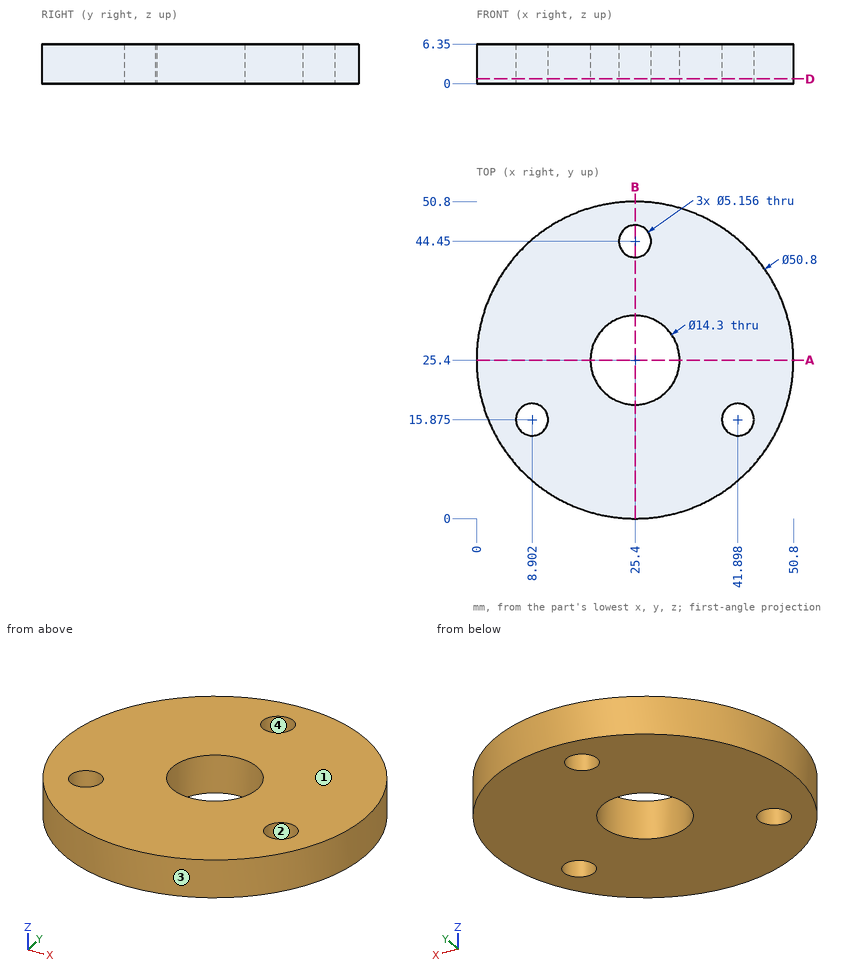
Job drawing, mm, ordinate dimensions from the low corner. One solid piece. Give positions to 0.01 mm unless a question says otherwise; leave off trailing zeros. Order: outer loops, then holes, each group sorted by start corner. A loop starts at its lowest first (then second) coordinate and runs counter-clockwise, first axis right, second up. Notation, with made-up numbers: M -8,59.25 L 25,59.25 A35 cw 25,96.25 Z; hole C 3,75 d5. An arc over 180 degrees is marked long. Put each result on its own line as item: value. Start each with the question number.
(1) Band-saw the part on B-B on x = 25.4. Give the cut face in (y, z), then the cut area to 3 significant figures.
(2) Drill centre lines: L1, parallel to Y at x = 25.4, z = 3.75; L2, parallel to X at y = 14, z = 3.5; L3, parallel to X at y = 30, z = 0.75 (1 decimal). Where is each one in solid material? Low to high. Write a range as [from, to].
(3) Band-saw the part on A-A on y = 25.4. Give the cut face in (x, z).
(4) Pin check, flat tips, straight feed: pin 1 Ø11.5 at (x, y) = (25.4, 25.4) entering from +Z; pin 2 Ø2 at (y, z) = (36, 4) entering from +X. Stop position of each tip, or through.
(5) Band-saw the part on D-D on z = 0.75. Count the separate pieces of the cut face and the enclosed holes in it, then the cut area to 3 significant figures.
(6) Pull direction Y, two halves, no side cores. Call the marked faces 1, 2, 3 and 4: released by +Y, released by -Y, zero draft, split by the parting line, or undercut.
Results below:
1. outline: M 0,0 L 18.25,0 L 18.25,6.35 L 0,6.35 Z; M 32.55,0 L 41.87,0 L 41.87,6.35 L 32.55,6.35 Z; M 47.03,0 L 50.8,0 L 50.8,6.35 L 47.03,6.35 Z
1. area: 199 mm2
2. L1: y = [0, 18.25], [32.55, 41.87], [47.03, 50.8]
2. L2: x = [2.7, 7.13], [10.67, 40.13], [43.67, 48.1]
2. L3: x = [0.4, 19.9], [30.9, 50.4]
3. outline: M 0,0 L 18.25,0 L 18.25,6.35 L 0,6.35 Z; M 32.55,0 L 50.8,0 L 50.8,6.35 L 32.55,6.35 Z
4. pin 1: passes through
4. pin 2: stops at x = 48.92
5. separate pieces: 1
5. enclosed holes: 4
5. area: 1,800 mm2
6. face 1: zero draft
6. face 2: undercut
6. face 3: split by the parting line
6. face 4: undercut
